For this review, take the finished solid that the model builds, in its own axes (mm). Face numbers are marked on the shaded views. A direction names the side the tool comes from. Coordinates: 2 decimals unless noted, no trailing zeros. Loops run counter-clockwise (first coordinate to the right, second up) from the corner with the lowest first, then second, coordinate; pieces in that order, holes last. Notation, with made-up numbers: M 49,0 L 99,0 A10 ccw 99,9 Z; hole C 7.5,6.25 d3. An arc over 180 degrees is marked long. Answer as a JSON object with one key per item and string values. Group by question number.
Item 1: Tool access review of the marked faces 1 and 2: name each direction out of +Z, -Z, +X, -X, +Y, -Y from which nothing blocks a thin tool from reaching the whole face with its end or side.
Item 2: Insertion check: pin 1 (3 mm diameter, centred on y = -2, z = 14, fed in from +X); pin 2 (1.5 mm diameter, centred on x = -1.5, z = 5.5, fed in from +Y). Each pin has a flat end and moves straight along its axis. Give the tip position at first contact, or say it passes through.
Item 3: Add section A-A (z = 11.5). State the section outline as (x, y) points.
Item 4: Wall thickness on L1, parallel to Z at x = -1, y = 3; L2, parallel to Y at x = 0.25, z = 6.25; L3, parallel to Z at x = 1.75, y = 0.5: over which ranges is each line inside the solid? List them lowest first. Write a range as from..to.
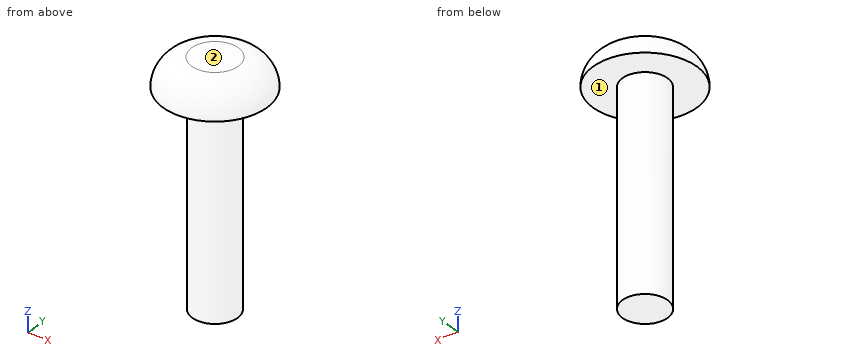
Autodesk Inventor part; units mm, degrees
ref_plane "YZ Plane" through (0, 0, 0) normal (1, 0, 0) x (0, 1, 0)
ref_plane "XZ Plane" through (0, 0, 0) normal (0, 1, 0) x (-1, 0, 0)
ref_plane "XY Plane" through (0, 0, 0) normal (0, 0, 1) x (1, 0, 0)
sketch "スケッチ1" plane through (0, 0, 0) normal (0, 0, 1) x (1, 0, 0)
  circle A0 centre (0, 0) radius 1.5
  dimension "d0" = 3
extrude "押し出し1" add sketch "スケッチ1" along normal blind 14
sketch "スケッチ2" plane through (0, 0, 14) normal (0, 0, 1) x (1, 0, 0)
  circle A0 centre (0, 0) radius 3.45
  dimension "d3" = 6.9
extrude "押し出し2" add sketch "スケッチ2" along normal blind 1.9
fillet "フィレット1" radius 1.9 1 edges at (-3.45, 0, 15.9)
thread "ねじ1"
properties part number "M3トラス頭ネジ　14" material "鉄 灰色"
From the geometry:
{
 "1": {"face 1": "-Z", "face 2": "+Z, +X, -X, +Y, -Y"},
 "2": {"pin 1": "stops at x = 3.41", "pin 2": "stops at y = 1.3"},
 "3": {"outline": "C 0,0 d3"},
 "4": {"L1": "z = 14..15.01", "L2": "y = -1.48..1.48", "L3": "z = 14..15.88"}
}
